```python
from build123d import *

# Parameters (mm, degrees)
F1_DEPTH = 3.175


# Not quite as in the source:
# - a feature names something its author has since deleted; it is built from what else it names


with BuildPart() as f1:
    # F0 (on Front) → F1 (new body, symmetric)
    with BuildSketch(Plane.XZ):
        Polygon((13.7837369962, 22.4047590313), (13.7837369962, -9.4272618645), (20.4636742089, -9.4272618645), (20.4636742089, -0.4338561879), (15.9735461484, 4.0562718726), (20.4636742089, 8.5463999331), (15.9735461484, 13.0365279937), (20.4636742089, 17.5266560542), (15.978414683, 22.0119155801), (20.4636742089, 26.497175106), (15.978414683, 30.9824346319), (20.4636742089, 35.4676941578), (15.9735461484, 39.9578222184), (20.4636742089, 44.4479502789), (20.4636742089, 49.9097465079), (13.7837369962, 49.9097465079), (13.7837369962, 26.6143454669), align=None)
        with BuildLine():
            ThreePointArc((1.5690815371, -26.4578800095), (2.166296426, -27.2647981392), (2.3779042983, -28.246126117))
            ThreePointArc((2.3779042983, -28.246126117), (2.2515693271, -29.011442898), (1.8859695789, -29.69555336))
            ThreePointArc((1.8859695789, -29.69555336), (15.116594907, -23.1743956519), (20.4636742089, -9.4272618645))
            Line((20.4636742089, -9.4272618645), (13.7837369962, -9.4272618645))
            ThreePointArc((13.7837369962, -9.4272618645), (10.4143723985, -19.9062857024), (1.5690815371, -26.4578800095))
        make_face()
        with BuildLine():
            Line((1.5079542983, 22.4047590313), (13.7837369962, 22.4047590313))
            Line((13.7837369962, 22.4047590313), (13.7837369962, 26.6143454669))
            Line((13.7837369962, 26.6143454669), (-0.0033457017, 26.6143454669))
            ThreePointArc((-0.0033457017, 26.6143454669), (1.6712163547, 25.9118815011), (2.363628681, 24.2331382585))
            ThreePointArc((2.363628681, 24.2331382585), (2.1391272177, 23.2237883133), (1.5079542983, 22.4047590313))
        make_face()
    extrude(amount=F1_DEPTH, both=True)


solid = f1.part
```
Can you work these out from the model? Positions are in its coordinate system, mm. A direction names the side the tool comes from. Give positions to 0.01 mm unless a question says otherwise; leave off trailing zeros. Loops run counter-clockwise (first coordinate to the right, second up) from the corner with the lowest first, then second, coordinate; pieces in that order, holes last. Notation, with made-up numbers: M 77.25,18.25 L 134.25,18.25 A30 cw 134.25,48.25 Z; hole C 69,50 d5. An arc over 180 degrees is marked long. Use CSV: the item, a comma, the result in double quotes. Start each with the question number.
1. Imagine slicing it at B-B, the plane x = 18.75. Write out the boundary of the cut face in (y, z) (1 decimal).
2. Imagine slicing it at A-A, the plane x = 11.5. Write out the boundary of the cut face in (y, z) (3 decimals), plus the area to 3 significant figures.
3. Imagine slicing it at C-C, the plane y = -1.25. Write out the boundary of the cut face in (x, z), plus the area to 3 significant figures.
4. If I drill on L1, parallel to Z at x = 17.25, y = 2.25; L2, parallel to Z at x = 18.75, y = 0; L3, parallel to Z at x = 7.5, y = -1.25, over which ranges is the centre line in solid material (lowest first)?
5. On a 3-axis mill with a long thin cutter (end or side, diameter ignored), from which of +Z, -Z, +X, -X, +Y, -Y can I reach the whole of each face in a straight line? I mean faces 1 (the face through (14, 3.175, 7)), 2 (the face through (10.505, -0.044, -19.779)), 3 (the face through (18.25, -0.04, 1.78)). Say none if no direction works.
6. For P1, Ø1, axis at x = 7, y = 2, coming from the +Z side; P2, Ø12, axis at x = 10.5, z = -19, coming from the +Y side (3 decimals); P3, Ø1.9, axis at y = -1, z = 5, coming from the -X side; P4, Ø1, axis at y = 0, z = 15.5, coming from the +X side, each with a flat end and sliding along its axis, tell me the tip position at first contact or that it passes through.
7. If we mould it in two halves opening along Z, with no side actions, what happens to faces 4 (the face through (20.464, 0, -5)), 5 (the face through (13.784, 0, 7)), 6 (the face through (15, 0, -23.3))? For each: released by +Z, released by -Z, zero draft, split by the parting line, or undercut.
8. Imagine slicing it at D-D, the plane z = -22. Write out the boundary of the cut face in (x, y) (3 decimals).
Response values:
1,outline,"M -3.2,-17.6 L 3.2,-17.6 L 3.2,1.3 L -3.2,1.3 Z; M -3.2,6.8 L 3.2,6.8 L 3.2,10.3 L -3.2,10.3 Z; M -3.2,15.8 L 3.2,15.8 L 3.2,19.2 L -3.2,19.2 Z; M -3.2,24.8 L 3.2,24.8 L 3.2,28.2 L -3.2,28.2 Z; M -3.2,33.8 L 3.2,33.8 L 3.2,37.2 L -3.2,37.2 Z; M -3.2,42.7 L 3.2,42.7 L 3.2,49.9 L -3.2,49.9 Z"
2,outline,"M -3.175,-26.291 L 3.175,-26.291 L 3.175,-18.197 L -3.175,-18.197 Z; M -3.175,22.405 L 3.175,22.405 L 3.175,26.614 L -3.175,26.614 Z"
2,area,"78.1 mm^2"
3,outline,"M 0,26.61 A2.38 cw 1.51,22.4 L 13.78,22.4 L 13.78,-9.43 A17.98 cw 1.57,-26.46 A2.38 cw 1.89,-29.7 A20.35 ccw 20.46,-9.43 L 20.46,-0.43 L 15.97,4.06 L 20.46,8.55 L 15.97,13.04 L 20.46,17.53 L 15.98,22.01 L 20.46,26.5 L 15.98,30.98 L 20.46,35.47 L 15.97,39.96 L 20.46,44.45 L 20.46,49.91 L 13.78,49.91 L 13.78,26.61 Z"
3,area,"487 mm^2"
4,L1,"-20.4 to 2.78, 5.33 to 11.76, 14.31 to 20.74, 23.28 to 29.71, 32.25 to 38.68, 41.23 to 49.91"
4,L2,"-17.6 to 1.28, 6.83 to 10.26, 15.81 to 19.24, 24.78 to 28.21, 33.75 to 37.18, 42.73 to 49.91"
4,L3,"-28.39 to -23.08, 22.4 to 26.61"
5,face 1,"+Z, -Z, +X, -X, +Y"
5,face 2,"-X, +Y, -Y"
5,face 3,"+X, +Y, -Y"
6,P1,"z = 26.61"
6,P2,"y = 3.175"
6,P3,"x = 13.78"
6,P4,"x = 18.94"
7,face 4,"zero draft"
7,face 5,"undercut"
7,face 6,"released by -Z"
8,outline,"M 8.657,-3.175 L 16.114,-3.175 L 16.114,3.175 L 8.657,3.175 Z"
